```python
from build123d import *

# Parameters (mm, degrees)
EXTRUDE_THIN1_DEPTH = 14.375
CHAMFER1_SIZE       = 0.508


with BuildPart() as part:
    # Sketch2 → Extrude-Thin1 (new, symmetric)
    with BuildSketch(Plane.XY):
        Polygon((0, 63.5), (-63.5, 63.5), (-63.5, 0), (-58.7375, 0), (-58.7375, 58.7375), (0, 58.7375), align=None)
    extrude(amount=EXTRUDE_THIN1_DEPTH, both=True)

    # Chamfer1
    chamfer1_edges = [part.edges().sort_by_distance(p)[0] for p in [
        (-63.5, 63.5, 0),
        (-58.7375, 58.7375, 0),
    ]]
    chamfer(chamfer1_edges, length=CHAMFER1_SIZE)

    # Mirror1: part across plane


with BuildPart() as part_1:
    add(part.part)
    add(part.part.mirror(Plane(origin=(0, 63.5, 14.375), x_dir=(0, 0, 1), z_dir=(1, 0, 0))))

    # Mirror2: part across plane


with BuildPart() as part_2:
    add(part_1.part)
    add(part_1.part.mirror(Plane(origin=(-58.7375, 0, 14.375), x_dir=(0, 0, 1), z_dir=(0, -1, 0))))


solid = part_2.part
```
Build history of the part. All positions in model axes, mm. A direction names the side the tool comes from. Coordinates: 2 decimals unless noted, no trailing zeros. Write each loop counter-clockwise with the first axis right and the second up, starting at its lowest first coordinate (ties: lowest second). Pieces come first, ordered by that corner, then holes.
1. Pull direction X, two halves, no side cores. Call faces 3 (the flat face through (-1, -63.5, 0)), 4 (the flat face through (63.5, -1, 0)), 5 (the flat face through (-58.738, 1, 0)), 6 (the flat face through (-63.5, -1, 0)): released by +X, released by -X, zero draft, split by the parting line, or undercut.
Answer block:
face 3: zero draft
face 4: released by +X
face 5: undercut
face 6: released by -X
2. Band-saw the part on A-A, the plane y = -52.5. Give the cut face in (x, z) (1 decimal), and give its area (3 significant figures).
Answer block:
outline: (-63.5, -14.4) - (-58.7, -14.4) - (-58.7, 14.4) - (-63.5, 14.4) - close; (58.7, -14.4) - (63.5, -14.4) - (63.5, 14.4) - (58.7, 14.4) - close
area: 274 mm2
3. Band-saw the part on B-B, the plane z = 10.75. Give the cut face in (x, y), and give its area (3 significant figures).
Answer block:
outline: (-63.5, -62.99) - (-62.99, -63.5) - (62.99, -63.5) - (63.5, -62.99) - (63.5, 62.99) - (62.99, 63.5) - (-62.99, 63.5) - (-63.5, 62.99) - close; hole (-58.74, -58.23) - (-58.23, -58.74) - (58.23, -58.74) - (58.74, -58.23) - (58.74, 58.23) - (58.23, 58.74) - (-58.23, 58.74) - (-58.74, 58.23) - close
area: 2,330 mm2
4. 3-axis set-ups, long thin cutter, end or side, ignore diameter. For faces 1 (the flat face through (-1, 63.5, 0)), 2 (the flat face through (58.738, 1, 0)): which of +Z, -Z, +X, -X, +Y, -Y reach the whole face in a straight line?
Answer block:
face 1: +Z, -Z, +X, -X, +Y
face 2: +Z, -Z
5. Drill centre line: probe 1 along Y at (x, z) = (-14, 0.5). Where is it in solid material? Low to high.
Answer block:
probe 1: y = -63.5 to -58.74, 58.74 to 63.5
